Can you work these out from the model? Positions are in its coordinate system, mm. Face numbers are marked on the shaded views. A direction names the side the tool comes from. Round coordinates to 2 decimals unless told otherwise and drop trailing zeros. Order: outer loops, then holes, each group sorted by start corner. A loop starts at its lowest first (then second) coordinate and runs counter-clockwise, first axis right, second up.
Q1. If we section it at A-A (x = -58.04): Please give me the cut outline in (y, z).
Q2. If we section it at B-B (x = 9.5): Please give me the cut outline in (y, z).
Q3. Will these pins go through, and if not, where does the flat tip stop? P1, Ø3, axis at y = -0.5, z = 7, coming from the +X side; P2, Ø3, axis at x = -65, z = 7, coming from the +Y side; P3, Ø2.5, axis at y = 0.5, z = 6, coming from the -X side.
Q4. We'd pull the mould along X, two halves only. Please class the marked faces 1, 2 and 3: pulls with the +X half, pulls with the -X half, needs draft (parallel to the pull), parting line crosses it, or undercut.
Q5. For the marked faces 4, 5 and 6, which set-ups out of +Z, -Z, +X, -X, +Y, -Y let a thin tool reach every point of the face, with its end or its side?
Q6. If I drill on line 1 (X direction, y = 9, z = 4.75); line 2 (X direction, y = -9.25, z = 7.5); line 3 (Y direction, x = -58.04, z = 12.25), over which ranges is the centre line in solid material (lowest first)?
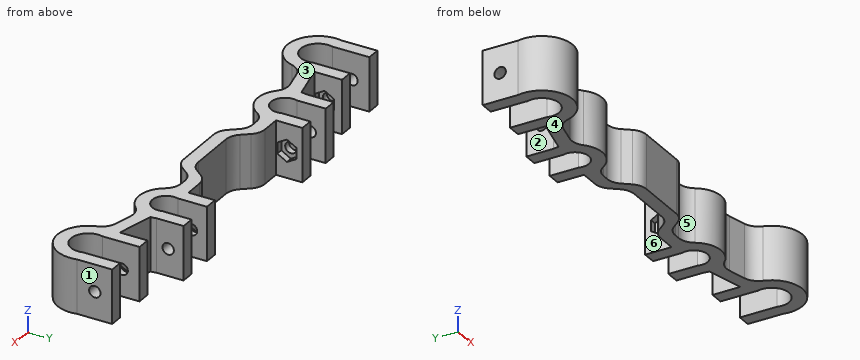
from build123d import *

# Parameters (mm, degrees)
F1_DEPTH = 16
F2_R     = 1.7
F3_DEPTH = 15.8
F4_DEPTH = 2
F5_R     = 1.7
F6_DEPTH = 17.8
F7_DEPTH = 2
F8_R     = 5


# Not quite as in the source:
# - a feature names something its author has since deleted; it is built from what else it names


with BuildPart() as f1:
    # F0 (on Top) → F1 (new body)
    with BuildSketch(Plane.XY):
        with BuildLine():
            ThreePointArc((-26.1, 1.2649110641), (-30, -4.1), (-33.9, 1.2649110641))
            Line((-33.9, 1.2649110641), (-33.9, 7.0992957397))
            ThreePointArc((-33.9, 7.0992957397), (-36.4699456608, 4.8733769756), (-37.9, 1.788854382))
            ThreePointArc((-37.9, 1.788854382), (-38.0425692419, 0.9628499311), (-38.0990116086, 0.1265344399))
            ThreePointArc((-38.0990116086, 0.1265344399), (-37.8794890645, -1.8771393349), (-37.1720292209, -3.7645712709))
            ThreePointArc((-37.1720292209, -3.7645712709), (-29.054976567, -8.0446833817), (-22.1507962187, -2))
            ThreePointArc((-22.1507962187, -2), (-21.9, 0), (-22.1507962187, 2))
            ThreePointArc((-22.1507962187, 2), (-23.5959659875, 4.9596722035), (-26.1, 7.0992957397))
            Line((-26.1, 7.0992957397), (-26.1, 1.2649110641))
        make_face()
        with BuildLine():
            ThreePointArc((-37.9, 1.788854382), (-36.4699456608, 4.8733769756), (-33.9, 7.0992957397))
            Line((-33.9, 7.0992957397), (-33.9, 9.8649110641))
            Line((-33.9, 9.8649110641), (-37.9, 9.8649110641))
            Line((-37.9, 9.8649110641), (-37.9, 1.788854382))
        make_face()
        with BuildLine():
            Line((-26.1, 9.8649110641), (-26.1, 7.0992957397))
            ThreePointArc((-26.1, 7.0992957397), (-23.5959659875, 4.9596722035), (-22.1507962187, 2))
            Line((-22.1507962187, 2), (-22.1, 2))
            Line((-22.1, 2), (-22.1, 9.8649110641))
            Line((-22.1, 9.8649110641), (-26.1, 9.8649110641))
        make_face()
        with BuildLine():
            Line((-22.1, 2), (-22.1507962187, 2))
            ThreePointArc((-22.1507962187, 2), (-21.9, 0), (-22.1507962187, -2))
            Line((-22.1507962187, -2), (-16.1507962187, -2))
            Line((-16.1507962187, -2), (-14.7945886775, -2))
            Line((-14.7945886775, -2), (-10, -8))
            Line((-10, -8), (0, -8))
            Line((0, -8), (0, -4))
            Line((0, -4), (-6, -4))
            Line((-6, -4), (-9.3562075412, -4))
            Line((-9.3562075412, -4), (-14.1507962187, 2))
            Line((-14.1507962187, 2), (-22.1, 2))
        make_face()
        with BuildLine():
            ThreePointArc((-37.1720292209, -3.7645712709), (-37.8794890645, -1.8771393349), (-38.0990116086, 0.1265344399))
            Line((-38.0990116086, 0.1265344399), (-49.14, -2.5037723523))
            Line((-49.14, -2.5037723523), (-49.14, -4.7826334039))
            ThreePointArc((-49.14, -4.7826334039), (-48.9961671585, -5.6705013446), (-48.9406864116, -6.5682314005))
            Line((-48.9406864116, -6.5682314005), (-37.1720292209, -3.7645712709))
        make_face()
        with BuildLine():
            Line((-49.14, -4.7826334039), (-49.14, -2.5037723523))
            Line((-49.14, -2.5037723523), (-49.8676687992, -2.6771256897))
            ThreePointArc((-49.8676687992, -2.6771256897), (-49.4391620268, -3.7075286109), (-49.14, -4.7826334039))
        make_face()
        with BuildLine():
            Line((-49.8676687992, -2.6771256897), (-49.14, -2.5037723523))
            Line((-49.14, -2.5037723523), (-49.14, 5.7342135624))
            Line((-49.14, 5.7342135624), (-53.14, 5.7342135624))
            Line((-53.14, 5.7342135624), (-53.14, 0.9881158051))
            ThreePointArc((-53.14, 0.9881158051), (-51.2517778793, -0.6194686338), (-49.8676687992, -2.6771256897))
        make_face()
        with BuildLine():
            ThreePointArc((-66.94, -4.7826334039), (-58.9383437694, -15.7355495952), (-48.9406864116, -6.5682314005))
            ThreePointArc((-48.9406864116, -6.5682314005), (-48.9961671585, -5.6705013446), (-49.14, -4.7826334039))
            ThreePointArc((-49.14, -4.7826334039), (-49.4391620268, -3.7075286109), (-49.8676687992, -2.6771256897))
            ThreePointArc((-49.8676687992, -2.6771256897), (-51.2517778793, -0.6194686338), (-53.14, 0.9881158051))
            Line((-53.14, 0.9881158051), (-53.14, -5.2657864376))
            ThreePointArc((-53.14, -5.2657864376), (-58.04, -11.78), (-62.94, -5.2657864376))
            Line((-62.94, -5.2657864376), (-62.94, 0.9881158051))
            ThreePointArc((-62.94, 0.9881158051), (-65.5189963637, -1.4959269496), (-66.94, -4.7826334039))
        make_face()
        with BuildLine():
            Line((-66.94, 5.7342135624), (-66.94, -4.7826334039))
            ThreePointArc((-66.94, -4.7826334039), (-65.5189963637, -1.4959269496), (-62.94, 0.9881158051))
            Line((-62.94, 0.9881158051), (-62.94, 5.7342135624))
            Line((-62.94, 5.7342135624), (-66.94, 5.7342135624))
        make_face()
    extrude(amount=F1_DEPTH)

    # F2 (on face) → F3 (cut, through all)
    with BuildSketch(Plane.YZ.offset(-22.1)):
        with Locations((5.2649110641, 8)):
            Circle(F2_R)
    extrude(amount=-F3_DEPTH, mode=Mode.SUBTRACT)

    # F2 (on face) → F4 (cut)
    with BuildSketch(Plane.YZ.offset(-22.1)):
        Polygon((8.1149110641, 6.3545517328), (8.1149110641, 9.6454482672), (5.2649110641, 11.2908965344), (2.4149110641, 9.6454482672), (2.4149110641, 6.3545517328), (5.2649110641, 4.7091034656), align=None)
        with Locations((5.2649110641, 8)):
            Circle(F2_R, mode=Mode.SUBTRACT)
    extrude(amount=-F4_DEPTH, mode=Mode.SUBTRACT)

    # F5 (on face) → F6 (cut, through all)
    with BuildSketch(Plane.YZ.offset(-49.14)):
        with Locations((0.5462276477, 8)):
            Circle(F5_R)
    extrude(amount=-F6_DEPTH, mode=Mode.SUBTRACT)

    # F5 (on face) → F7 (cut)
    with BuildSketch(Plane.YZ.offset(-49.14)):
        Polygon((3.3962276477, 6.3545517328), (3.3962276477, 9.6454482672), (0.5462276477, 11.2908965344), (-2.3037723523, 9.6454482672), (-2.3037723523, 6.3545517328), (0.5462276477, 4.7091034656), align=None)
        with Locations((0.5462276477, 8)):
            Circle(F5_R, mode=Mode.SUBTRACT)
    extrude(amount=-F7_DEPTH, mode=Mode.SUBTRACT)

    # F8
    f8_edges = [f1.edges().sort_by_distance(p)[0] for p in [
        (-48.940686, -6.568231, 8),
        (-37.172029, -3.764571, 8),
        (-22.150796, -2, 8),
        (-14.794589, -2, 8),
        (-10, -8, 8),
        (-9.356208, -4, 8),
        (-14.150796, 2, 8),
    ]]
    fillet(f8_edges, radius=F8_R)

    # F9: F1 across plane


with BuildPart() as f1_1:
    add(f1.part)
    add(f1.part.mirror(Plane.YZ))


solid = f1_1.part
Solution:
1. outline: (-15.78, 0) - (-11.78, 0) - (-11.78, 16) - (-15.78, 16) - close
2. outline: (-7.62, 0) - (-3.3, 0) - (-3.3, 16) - (-7.62, 16) - close
3. P1: stops at x = 66.94
3. P2: stops at y = 5.73
3. P3: stops at x = -66.94
4. face 1: pulls with the +X half
4. face 2: undercut
4. face 3: needs draft
5. face 4: -Z, +X, -X, +Y, -Y
5. face 5: +Z, -Z, -Y
5. face 6: +Z, -Z, +Y
6. line 1: x = -37.9 to -33.9, -26.1 to -22.1, 22.1 to 26.1, 33.9 to 37.9
6. line 2: x = -66.77 to -62.45, -53.63 to -49.31, 49.31 to 53.63, 62.45 to 66.77
6. line 3: y = -15.78 to -11.78
